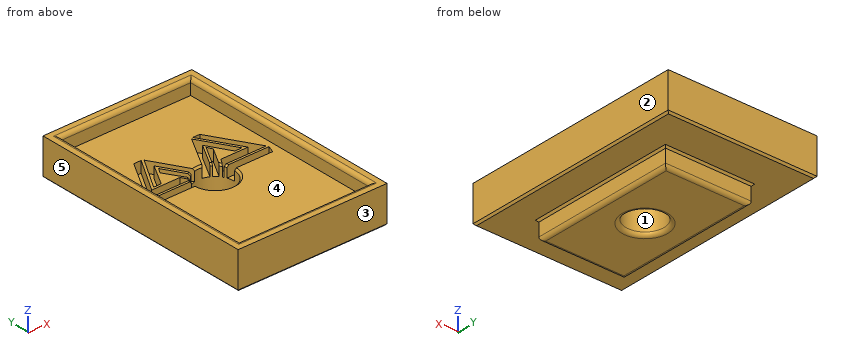
```python
from build123d import *

# Parameters (mm, degrees)
SKETCH1_W           = 20
SKETCH1_H           = 30
BOSS_EXTRUDE1_DEPTH = 5
SKETCH4_W           = 11.5
SKETCH4_H           = 19.5
BOSS_EXTRUDE2_DEPTH = 2.5
SKETCH2_R           = 2.55
CUT_EXTRUDE1_DEPTH  = 8.5
SKETCH3_W           = 17.5
SKETCH3_H           = 27.5
CUT_EXTRUDE2_DEPTH  = 2
FILLET1_R           = 0.5
CHAMFER1_SIZE       = 0.25
CHAMFER2_SIZE       = 0.25
FILLET2_R           = 0.5
CUT_EXTRUDE5_DEPTH  = 3.5


with BuildPart() as part:
    # Sketch1 → Boss-Extrude1 (new body)
    with BuildSketch(Plane.XY):
        Rectangle(SKETCH1_W, SKETCH1_H)
    extrude(amount=BOSS_EXTRUDE1_DEPTH)

    # Sketch4 → Boss-Extrude2 (add)
    with BuildSketch(Plane(origin=(0, 0, 0), x_dir=(-1, 0, 0), z_dir=(0, 0, -1))):
        Rectangle(SKETCH4_W, SKETCH4_H)
    extrude(amount=BOSS_EXTRUDE2_DEPTH)

    # Sketch2 → Cut-Extrude1 (cut, through all)
    with BuildSketch(Plane.XY.offset(5)):
        Circle(SKETCH2_R)
    extrude(amount=-CUT_EXTRUDE1_DEPTH, mode=Mode.SUBTRACT)

    # Sketch3 → Cut-Extrude2 (cut)
    with BuildSketch(Plane.XY.offset(5)):
        Rectangle(SKETCH3_W, SKETCH3_H)
    extrude(amount=-CUT_EXTRUDE2_DEPTH, mode=Mode.SUBTRACT)

    # Fillet1
    fillet1_edges = [part.edges().sort_by_distance(p)[0] for p in [
        (-5.75, 0, -2.5),
        (0, 9.75, -2.5),
        (5.75, 0, -2.5),
        (0, -9.75, -2.5),
        (-2.55, 0, -2.5),
    ]]
    fillet(fillet1_edges, radius=FILLET1_R)

    # Chamfer1
    chamfer1_edges = [part.edges().sort_by_distance(p)[0] for p in [
        (-5.75, 0, 0),
        (0, 9.75, 0),
        (5.75, 0, 0),
        (0, -9.75, 0),
        (0, -15, 0),
        (-10, 0, 0),
        (0, 15, 0),
        (10, 0, 0),
    ]]
    chamfer(chamfer1_edges, length=CHAMFER1_SIZE)

    # Chamfer2
    chamfer2_edges = [part.edges().sort_by_distance(p)[0] for p in [
        (-2.55, 0, 3),
    ]]
    chamfer(chamfer2_edges, length=CHAMFER2_SIZE)

    # Fillet2
    fillet2_edges = [part.edges().sort_by_distance(p)[0] for p in [
        (8.75, 0, 5),
        (0, 13.75, 5),
        (-8.75, 0, 5),
        (0, -13.75, 5),
    ]]
    fillet(fillet2_edges, radius=FILLET2_R)

    # Mobious Logo → Cut-Extrude5 (cut)
    with BuildSketch(Plane(origin=(0, 0, 5), x_dir=(-1, 0, 0), z_dir=(0, 0, 1))):
        Polygon((3.509190245, -7.338202372), (4.502229849, -7.338202372), (8.08727113, -1.177990592), (2.246851765, -1.177990592), (2.773304458, -2.208730349), (6.572464955, -2.208730349), align=None)
        Polygon((3.694333222, -4.224434122), (3.239891369, -4.96500603), (0.344928456, 0.101179067), (7.868465794, 0.101179067), (8.091043636, -0.891860536), (1.68474111, -0.891860536), align=None)
        Polygon((6.050698383, -2.50765379), (3.239891369, -7.186721754), (0.041967221, -1.598400594), (-3.139125747, -7.186721754), (-5.816728556, -2.50765379), (-4.85985244, -2.50765379), (-3.139125747, -5.514596088), (0, 0), (3.239891369, -5.661658206), (5.035275167, -2.50765379), align=None)
        Polygon((-3.425255803, -7.338202372), (-4.367801867, -7.338202372), (-7.91918079, -1.177990592), (-2.061930245, -1.177990592), (-2.718346254, -2.208730349), (-6.370712255, -2.208730349), align=None)
        Polygon((-3.139125747, -4.96500603), (-0.227331655, 0.101179067), (-7.649881914, 0.101179067), (-8.043673481, -0.891860536), (-1.556994853, -0.891860536), (-3.494124276, -4.262241786), align=None)
    extrude(amount=-CUT_EXTRUDE5_DEPTH, mode=Mode.SUBTRACT)


solid = part.part
```
Input: part model. Units: mm. Frame: model coordinates. Face numbers are marked on the shaded views. A direction names the side the tool comes from. Coordinates: 2 decimals unless noted, no trailing zeros. Write each loop counter-clockwise with the first axis right and the second up, starting at its lowest first coordinate (ties: lowest second). Pieces come first, ordered by that corner, then holes. Notation, with made-up numbers: (-11, 86) - (9, 86) arc R26 ccw to (9, 110) - close; hole circle Ø10 at (28.5, -17.5). An arc over 180 degrees is marked (long way). Put each result on its own line as item: value. Start each with the question number.
1) Cut plane C-C (y = -3.5). Return the cut outline in (x, z).
2) Ray query, L1, parallel to X at y = 0, z = 0.7; L2, parallel to Y at x = 0, z = -0.35; L3, parallel to X at y = 0, z = -0.85. Return the intervals inside material, ascending.
3) Cut plane D-D (x = -7.25). Return the cut outline in (y, z), plus the area to 3 significant figures.
4) Contact query for flat-ended pins moving along their axis: pin 1 (1.7 mm diameter, centred on x = -2.5, y = 3, fed in from +Z); pin 2 (0.9 mm diameter, centred on y = -3.5, z = -1.5, fed in from +X); pin 3 (2 mm diameter, centred on y = 6, z = -0.5, fed in from +X); pin 4 (1.9 mm diameter, centred on x = -1.5, z = -1.5, fed in from +Y). Output: stop coordinate, or through.
5) Cut plane B-B (z = 3.5). Return the cut outline in (x, y).
6) Cut plane A-A (x = 0). Return the cut outline in (y, z), plus the area to 3 significant figures.
7) Reachability of the marked faces 4 and 5 from +Z, -Z, +X, -X, +Y, -Y: full face, straight path, thin tool, end or side. Return the list, or none.
8) Mould query, pull axis X, two halves, no side actions, for the marked faces 1, 2 and 3. Classes: pulls with the +X half, pulls with the -X half, needs draft (parallel to the pull), parting line crosses it, or undercut.
Resolved:
1. outline: (-10, 0.25) - (-9.75, 0) - (-6, 0) - (-5.75, -0.25) - (-5.75, -2) arc R0.5 ccw to (-5.25, -2.5) - (5.25, -2.5) arc R0.5 ccw to (5.75, -2) - (5.75, -0.25) - (6, 0) - (9.75, 0) - (10, 0.25) - (10, 5) - (9.25, 5) arc R0.5 ccw to (8.75, 4.5) - (8.75, 3) - (-8.75, 3) - (-8.75, 4.5) arc R0.5 ccw to (-9.25, 5) - (-10, 5) - close
2. L1: x = -10 to -2.55, 2.55 to 10
2. L2: y = -9.75 to -2.55, 2.55 to 9.75
2. L3: x = -5.75 to -2.55, 2.55 to 5.75
3. outline: (-15, 0.25) - (-14.75, 0) - (14.75, 0) - (15, 0.25) - (15, 5) - (14.25, 5) arc R0.5 ccw to (13.75, 4.5) - (13.75, 3) - (2.62, 3) - (2.62, 1.5) - (1.18, 1.5) - (1.18, 3) - (0.89, 3) - (0.89, 1.5) - (-0.1, 1.5) - (-0.1, 3) - (-13.75, 3) - (-13.75, 4.5) arc R0.5 ccw to (-14.25, 5) - (-15, 5) - close
3. area: 91.2 mm2
4. pin 1: stops at z = 3
4. pin 2: stops at x = 5.75
4. pin 3: stops at x = 10
4. pin 4: stops at y = 9.75
5. outline: (-10, -15) - (10, -15) - (10, 15) - (-10, 15) - close; hole (-8.75, -13.75) - (8.75, -13.75) - (8.75, 13.75) - (-8.75, 13.75) - close
6. outline: (-15, 0.25) - (-14.75, 0) - (-10, 0) - (-9.75, -0.25) - (-9.75, -2) arc R0.5 ccw to (-9.25, -2.5) - (-3.05, -2.5) arc R0.5 ccw to (-2.55, -2) - (-2.55, 2.75) - (-2.8, 3) - (-13.75, 3) - (-13.75, 4.5) arc R0.5 ccw to (-14.25, 5) - (-15, 5) - close; (2.55, -2) arc R0.5 ccw to (3.05, -2.5) - (9.25, -2.5) arc R0.5 ccw to (9.75, -2) - (9.75, -0.25) - (10, 0) - (14.75, 0) - (15, 0.25) - (15, 5) - (14.25, 5) arc R0.5 ccw to (13.75, 4.5) - (13.75, 3) - (2.8, 3) - (2.55, 2.75) - close
6. area: 115 mm2
7. face 4: +Z
7. face 5: +Z, -Z, -X, +Y, -Y
8. face 1: undercut
8. face 2: pulls with the +X half
8. face 3: needs draft
